from build123d import *

# Parameters (mm, degrees)
ESQUISSE1_W             = 160
ESQUISSE1_H             = 68
ESQUISSE1_R             = 2.5
BOSS_EXTRU_1_DEPTH      = 12
ESQUISSE2_R             = 2.25
ENL_V_MAT_EXTRU_1_DEPTH = 15
ESQUISSE3_R             = 4.5
ENL_V_MAT_EXTRU_2_DEPTH = 5


with BuildPart() as part:
    # Esquisse1 → Boss.-Extru.1 (new body)
    with BuildSketch(Plane.XY):
        with Locations((80, 34)):
            Rectangle(ESQUISSE1_W, ESQUISSE1_H)
        with Locations((62.5, 39.5)):
            Circle(ESQUISSE1_R, mode=Mode.SUBTRACT)
        with Locations((32.5, 39.5)):
            Circle(ESQUISSE1_R, mode=Mode.SUBTRACT)
        with Locations((32.5, 7.5)):
            Circle(ESQUISSE1_R, mode=Mode.SUBTRACT)
        with Locations((62.5, 7.5)):
            Circle(ESQUISSE1_R, mode=Mode.SUBTRACT)
        with Locations(Location((97.5, 7.5, 0), (0, 0, 180))):
            Circle(ESQUISSE1_R, mode=Mode.SUBTRACT)
        with Locations(Location((127.5, 7.5, 0), (0, 0, 180))):
            Circle(ESQUISSE1_R, mode=Mode.SUBTRACT)
        with Locations(Location((127.5, 39.5, 0), (0, 0, 180))):
            Circle(ESQUISSE1_R, mode=Mode.SUBTRACT)
        with Locations(Location((97.5, 39.5, 0), (0, 0, 180))):
            Circle(ESQUISSE1_R, mode=Mode.SUBTRACT)
    extrude(amount=BOSS_EXTRU_1_DEPTH)

    # Esquisse2 → Enlèv. mat.-Extru.1 (cut)
    with BuildSketch(Plane(origin=(0, 68, 0), x_dir=(1, 0, 0), z_dir=(0, 1, 0))):
        with Locations(Location((15, -6, 0), (0, 0, 270))):
            Circle(ESQUISSE2_R)
        with Locations(Location((80, -6, 0), (0, 0, 270))):
            Circle(ESQUISSE2_R)
        with Locations(Location((145, -6, 0), (0, 0, 270))):
            Circle(ESQUISSE2_R)
    extrude(amount=-ENL_V_MAT_EXTRU_1_DEPTH, mode=Mode.SUBTRACT)

    # Esquisse3 → Enlèv. mat.-Extru.2 (cut)
    with BuildSketch(Plane(origin=(0, 0, 0), x_dir=(-1, 0, 0), z_dir=(0, 0, -1))):
        with Locations((-127.5, 39.5)):
            Circle(ESQUISSE3_R)
        with Locations((-127.5, 7.5)):
            Circle(ESQUISSE3_R)
        with Locations((-97.5, 39.5)):
            Circle(ESQUISSE3_R)
        with Locations((-62.5, 39.5)):
            Circle(ESQUISSE3_R)
        with Locations((-97.5, 7.5)):
            Circle(ESQUISSE3_R)
        with Locations((-62.5, 7.5)):
            Circle(ESQUISSE3_R)
        with Locations((-32.5, 7.5)):
            Circle(ESQUISSE3_R)
        with Locations((-32.5, 39.5)):
            Circle(ESQUISSE3_R)
    extrude(amount=-ENL_V_MAT_EXTRU_2_DEPTH, mode=Mode.SUBTRACT)


solid = part.part
Could you check a few things on this model? Use its own coordinates, in mm. A direction names the side the tool comes from. Give positions to 0.01 mm unless a question says otherwise; leave off trailing zeros. Loops run counter-clockwise (first coordinate to the right, second up) from the corner with the lowest first, then second, coordinate; pieces in that order, holes last. Notation, with made-up numbers: (26.5, 64) -> (48.5, 64) arc R13 cw to (48.5, 68) -> close; hole circle Ø7 at (27, -16.5). An arc over 180 degrees is marked (long way). Return JSON: item names as keys, results as strings.
Item 1: We'd pull the mould along Z, two halves only. Please class faces 4 (the flat face through (60.6, 5.6, 5)), 5 (the cylindrical face through (77.804, 60.605, 5.512)), 6 (the cylindrical face through (101.1, 36.8, 2.5)): +Z half, -Z half, draft (parallel to the pull), parting line (faces both ways), or undercut.
Geometry results:
{"face 4": "-Z half", "face 5": "undercut", "face 6": "draft"}
Item 2: If we section it at B-B on z = 1.5: Count the separate pieces of the cut face and the enclosed holes in it, plus the area to 3 significant figures.
Geometry results:
{"separate pieces": "1", "enclosed holes": "8", "area": "10,400 mm²"}
Item 3: I'm going to push a flat-ended pin straight in: pin 1 (4.5 mm diameter, centred on x = 128, y = 39, fed in from -Z). Where does the tip first touch, or does it pass through?
Geometry results:
{"pin 1": "stops at z = 5"}
Item 4: If we section it at A-A on x = 32.5: List the corners of the cut face in (y, z) for me.
Geometry results:
{"outline": "(0, 0) -> (3, 0) -> (3, 5) -> (5, 5) -> (5, 12) -> (0, 12) -> close; (10, 5) -> (12, 5) -> (12, 0) -> (35, 0) -> (35, 5) -> (37, 5) -> (37, 12) -> (10, 12) -> close; (42, 5) -> (44, 5) -> (44, 0) -> (68, 0) -> (68, 12) -> (42, 12) -> close"}
Item 5: I need wall thicknesses on L1, parallel to X at y = 39.5, z = 7; L2, parallel to Y at x = 127.5, z = 3.1; L3, parallel to Y at x = 62.5, z = 9.75. Which ranges of each line are inside material? Lowest first, please. Write a range as from..to.
Geometry results:
{"L1": "x = 0..30, 35..60, 65..95, 100..125, 130..160", "L2": "y = 0..3, 12..35, 44..68", "L3": "y = 0..5, 10..37, 42..68"}
Item 6: If we section it at D-D on x = 145: List the corners of the cut face in (y, z) for me.
Geometry results:
{"outline": "(0, 0) -> (68, 0) -> (68, 3.75) -> (53, 3.75) -> (53, 8.25) -> (68, 8.25) -> (68, 12) -> (0, 12) -> close"}
Item 7: Which directions (+Z, -Z, +X, -X, +Y, -Y) give clear straight access to the entire face, cutting with the end or side of a thin tool? Please do faces 1 (the cylindrical face through (28.208, 8.852, 2.465)), 2 (the flat face through (145, 53, 6)), 3 (the cylindrical face through (125.115, 6.749, 8.451)).
Geometry results:
{"face 1": "-Z", "face 2": "+Y", "face 3": "+Z, -Z"}
